Here's how the part is built. I have some questions about the finished solid (model axes, mm). A direction names the side the tool comes from. Coordinates: 2 decimals unless noted, no trailing zeros. Write each loop counter-clockwise with the first axis right and the second up, starting at its lowest first coordinate (ties: lowest second). Pieces come first, ordered by that corner, then holes.
(1) Thinking about a two-plate mould opening in Z: for faces 1 (the flat face through (-22, -2, -3)), 2 (the flat face through (50, -2, 12)), 3 (the flat face through (55, -2, -14)), which applies, released by +Z, released by -Z, zero draft, split by the parting line, or undercut?
(2) Which directions (+Z, -Z, +X, -X, +Y, -Y) give clear straight access to the entire face, cutting with the end or side of a thin tool? Please do faces 4 (the flat face through (-55, -2, 13)), 5 (the flat face through (-70, -2, -12)), 6 (the flat face through (-65, -2, 13)).
(3) Imagine slicing it at D-D, the plane y = -1.5. State how many separate pieces and enclosed holes the cut face has, plus the area to 3 significant figures.
(4) Imagine slicing it at C-C, the plane z = 0.5. List the corners of the cut face in (x, y) for me, plus the area to 3 significant figures.
(5) Imagine slicing it at B-B, the plane x = 10. List the corners of the cut face in (y, z) for me.
(6) Please list where these lines run through material, in increasing order: probe 1 along X at (y, z) = (-2.2, -2.75); probe 2 along X at (y, z) = (-0.8, 1.75); probe 3 along X at (y, z) = (-0.3, 1).
(7) For pin 1 Ø0.9 at (y, z) = (-1, 14) entering from -X; pin 2 Ø10 at (x, z) = (-20.5, 0) entering from -Y; pin 3 Ø0.9 at (x, y) = (72, -1.5) entering from -Z; pin 4 Ø0.9 at (x, y) = (-48.5, -1.5) entering from +Z, each with a flat end and sliding along its axis, tell me the tip position at first contact or that it passes through.
(8) Imagine slicing it at A-A, the plane z = 9.5. List the corners of the cut face in (x, y) for me, plus the area to 3 significant figures.
```python
from build123d import *

# Parameters (mm, degrees)
F0_W     = 151
F0_H     = 30
F1_DEPTH = 3
F2_W     = 5
F2_H     = 3
F2_W_2   = 6.448428
F2_W_3   = 10
F2_W_4   = 3.551572
F2_R     = 4.5
F2_R_2   = 1.5
F2_R_3   = 1.75
F2_R_4   = 3
F2_H_2   = 7
F3_DEPTH = 25


with BuildPart() as f1:
    # F0 (on Front) → F1 (new body)
    with BuildSketch(Plane.XZ):
        Rectangle(F0_W, F0_H)
    extrude(amount=F1_DEPTH)

    # F2 (on face) → F3 (cut)
    with BuildSketch(Plane.XZ.offset(3)):
        with Locations((-72.5, -13.5)):
            Rectangle(F2_W, F2_H)
        with Locations((-78.224214, -13.5)):
            Rectangle(F2_W_2, F2_H)
        with Locations((-67.5, -13.5)):
            Rectangle(F2_W, F2_H)
        with Locations((-72.5, 13.5)):
            Rectangle(F2_W, F2_H)
        with Locations((-78.224214, 13.5)):
            Rectangle(F2_W_2, F2_H)
        with Locations((-67.5, 13.5)):
            Rectangle(F2_W, F2_H)
        with Locations((-50, -13.5)):
            Rectangle(F2_W_3, F2_H)
        with Locations((-50, 13.5)):
            Rectangle(F2_W_3, F2_H)
        with Locations((-30, -13.5)):
            Rectangle(F2_W_3, F2_H)
        with Locations((-30, 13.5)):
            Rectangle(F2_W_3, F2_H)
        with Locations((-10, -13.5)):
            Rectangle(F2_W_3, F2_H)
        with Locations((-10, 13.5)):
            Rectangle(F2_W_3, F2_H)
        with Locations((10, -13.5)):
            Rectangle(F2_W_3, F2_H)
        with Locations((10, 13.5)):
            Rectangle(F2_W_3, F2_H)
        with Locations((30, -13.5)):
            Rectangle(F2_W_3, F2_H)
        with Locations((30, 13.5)):
            Rectangle(F2_W_3, F2_H)
        with Locations((50, -13.5)):
            Rectangle(F2_W_3, F2_H)
        with Locations((50, 13.5)):
            Rectangle(F2_W_3, F2_H)
        with Locations((66.775786, -13.5)):
            Rectangle(F2_W_4, F2_H)
        with Locations((71.775786, -13.5)):
            Rectangle(F2_W_2, F2_H)
        with Locations((77.5, -13.5)):
            Rectangle(F2_W, F2_H)
        with Locations((66.775786, 13.5)):
            Rectangle(F2_W_4, F2_H)
        with Locations((71.775786, 13.5)):
            Rectangle(F2_W_2, F2_H)
        with Locations((77.5, 13.5)):
            Rectangle(F2_W, F2_H)
        with Locations((9.295744, 0.5)):
            Circle(F2_R)
        with Locations((-11.304256, 9.5)):
            Circle(F2_R_2)
        with Locations((-11.304256, -8)):
            Circle(F2_R_3)
        with Locations((-2.204256, 0.5)):
            Circle(F2_R_4)
        with Locations((-22.204256, 0.5)):
            Rectangle(F2_W, F2_H_2)
    extrude(amount=-F3_DEPTH, mode=Mode.SUBTRACT)


solid = f1.part
```
Recorded:
1. face 1: undercut
1. face 2: released by +Z
1. face 3: zero draft
2. face 4: +Z, +Y, -Y
2. face 5: -Z, -X, +Y, -Y
2. face 6: +Z, -X, +Y, -Y
3. separate pieces: 1
3. enclosed holes: 5
3. area: 3,900 mm2
4. outline: (-75.5, -3) - (-24.7, -3) - (-24.7, 0) - (-75.5, 0) - close; (-19.7, -3) - (-5.2, -3) - (-5.2, 0) - (-19.7, 0) - close; (0.8, -3) - (4.8, -3) - (4.8, 0) - (0.8, 0) - close; (13.8, -3) - (75.5, -3) - (75.5, 0) - (13.8, 0) - close
4. area: 393 mm2
5. outline: (-3, -12) - (0, -12) - (0, -3.94) - (-3, -3.94) - close; (-3, 4.94) - (0, 4.94) - (0, 12) - (-3, 12) - close
6. probe 1: x = -75.5 to -24.7, -19.7 to 6.18, 12.41 to 75.5
6. probe 2: x = -75.5 to -24.7, -19.7 to -4.93, 0.52 to 4.97, 13.62 to 75.5
6. probe 3: x = -75.5 to -24.7, -19.7 to -5.16, 0.75 to 4.82, 13.77 to 75.5
7. pin 1: stops at x = -65
7. pin 2: stops at y = -3
7. pin 3: stops at z = -12
7. pin 4: stops at z = 12
8. outline: (-75.5, -3) - (-12.8, -3) - (-12.8, 0) - (-75.5, 0) - close; (-9.8, -3) - (75.5, -3) - (75.5, 0) - (-9.8, 0) - close
8. area: 444 mm2
